from build123d import *

# Parameters (mm, degrees)
MODEL_R                 = 1.600279216
MODEL_R_2               = 1.7
SALIENTE_EXTRUIR2_DEPTH = 3


with BuildPart() as part:
    # Model → Saliente-Extruir2 (new body)
    with BuildSketch(Plane.XY):
        with BuildLine():
            Line((271.351226454, 245.262259879), (270.71262235, 244.623655775))
            Line((270.71262235, 244.623655775), (270.71262235, 230.233550186))
            ThreePointArc((270.71262235, 230.233550186), (271.151962178, 229.172890015), (272.21262235, 228.733550186))
            Line((272.21262235, 228.733550186), (350.217232207, 228.733550186))
            ThreePointArc((350.217232207, 228.733550186), (351.277892379, 229.172890015), (351.717232207, 230.233550186))
            Line((351.717232207, 230.233550186), (351.717232207, 299.235954421))
            ThreePointArc((351.717232208, 299.235954421), (351.277892379, 300.296614592), (350.217232207, 300.735954421))
            Line((350.217232207, 300.735954421), (272.21262235, 300.735954421))
            ThreePointArc((272.21262235, 300.735954421), (271.151962178, 300.296614592), (270.71262235, 299.235954421))
            Line((270.71262235, 299.235954421), (270.71262235, 284.103268217))
            Line((270.71262235, 284.103268217), (271.351226454, 283.464664113))
            Line((271.351226454, 283.464664113), (271.97853318, 283.464664113))
            Line((271.97853318, 283.464664113), (272.77853318, 284.264664113))
            Line((272.77853318, 284.264664113), (276.051226454, 284.264664113))
            Line((276.051226454, 284.264664113), (276.251226454, 284.464664114))
            Line((276.251226454, 284.464664114), (276.251226454, 285.894852324))
            ThreePointArc((276.251226454, 285.894852324), (273.443758266, 287.176917482), (276.239508411, 288.48433854))
            Line((276.239508411, 288.48433854), (276.239508411, 294.917021597))
            ThreePointArc((276.239508411, 294.917021597), (273.696009795, 296.507802753), (276.661013605, 296.964664113))
            Line((276.661013605, 296.964664113), (279.851226454, 296.964664113))
            Line((279.851226454, 296.964664113), (281.651226454, 298.764664113))
            Line((281.651226454, 298.764664113), (341.055836311, 298.764664113))
            Line((341.055836311, 298.764664113), (342.855836311, 296.964664113))
            Line((342.855836311, 296.964664113), (345.9273642, 296.964664113))
            ThreePointArc((345.9273642, 296.964664113), (348.738416986, 297.034405979), (347.268369224, 294.637357529))
            Line((347.268369224, 294.637357529), (347.268369224, 288.812692031))
            ThreePointArc((347.268369224, 288.812692031), (348.543864828, 285.912196427), (345.643369224, 287.187692032))
            Line((345.643369224, 287.187692032), (344.134568969, 287.187692032))
            Line((344.134568969, 287.187692032), (344.134568969, 285.564664113))
            Line((344.134568969, 285.564664113), (344.934568969, 284.764664113))
            Line((344.934568969, 284.764664113), (349.36625565, 284.764664113))
            Line((349.36625565, 284.764664113), (349.86625565, 284.264664113))
            Line((349.86625565, 284.264664113), (349.86625565, 247.072679218))
            Line((349.86625565, 247.072679218), (348.055836311, 245.262259879))
            Line((348.055836311, 245.262259879), (344.855836311, 245.262259879))
            Line((344.855836311, 245.262259879), (344.468087014, 244.877634885))
            Line((344.468087014, 244.877634885), (344.468087014, 231.262259879))
            Line((344.468087014, 231.262259879), (343.968087014, 230.762259879))
            Line((343.968087014, 230.762259879), (278.151226454, 230.762259879))
            Line((278.151226454, 230.762259879), (277.651226454, 231.262259879))
            Line((277.651226454, 231.262259879), (277.651226454, 244.762259879))
            Line((277.651226454, 244.762259879), (277.151226454, 245.262259879))
            Line((277.151226454, 245.262259879), (271.351226454, 245.262259879))
        make_face()
        with Locations((275.263424864, 233.182413169)):
            Circle(MODEL_R, mode=Mode.SUBTRACT)
        with Locations((275.263424864, 242.182078667)):
            Circle(MODEL_R_2, mode=Mode.SUBTRACT)
        with Locations((347.268369224, 233.182413169)):
            Circle(MODEL_R, mode=Mode.SUBTRACT)
        with Locations((347.268369224, 242.182078667)):
            Circle(MODEL_R_2, mode=Mode.SUBTRACT)
    extrude(amount=SALIENTE_EXTRUIR2_DEPTH)


solid = part.part
Can you work these out from the model? Positions are in its coordinate system, mm. A direction names the side the tool comes from. Give positions to 0.01 mm unless a question says otherwise; leave off trailing zeros. Write each loop counter-clockwise with the first axis right and the second up, starting at its lowest first coordinate (ties: lowest second). Pieces come first, ordered by that corner, then holes. Notation, with made-up numbers: M -21.75,3.25 L 36.25,3.25 A18 cw 36.25,29.25 Z; hole C -23,1.25 d5. An arc over 180 degrees is marked long. Answer in a Markdown table with one row per item. Add a question column.
Item 1: Please list where these lines run through material, in increasing order: L1, parallel to Y at x = 302, z = 1.9; L2, parallel to X at y = 286.5, z = 1.65; L3, parallel to Y at x = 342, z = 0.6.
Item 2: We'd pull the mould along X, two halves only. Please class faces 4 (the flat face through (344.468, 238, 1)), 5 (the flat face through (277.651, 238, 1)), 6 (the flat face through (348.974, 246.18, 1.479)), 7 (the flat face through (274, 245.262, 1)): released by +X, released by -X, zero draft, split by the parting line, or undercut.
Item 3: Imagine slicing it at C-C, the plane z = 0.8. State how many separate pieces and enclosed holes the cut face has, plus the area to 3 significant figures.
Item 4: For pin 1 Ø5 at (x, y) = (347.35, 296.24) entering from +Z, with a flat end and sliding along its axis, tell me the tip position at first contact or that it passes through.
Item 5: Imagine slicing it at B-B, the plane y = 267.5. Write out the boundary of the cut face in (x, z).
Item 6: On a 3-axis mill with a long thin cutter (end or side, diameter ignored), from which of +Z, -Z, +X, -X, +Y, -Y can I reach the whole of each face in a straight line? I mean faces 1 (the flat face through (280.739, 297.852, 1.479)), 2 (the flat face through (346, 245.262, 1)), 3 (the flat face through (270.713, 292, 1)). Say none if no direction works.
Item 7: Imagine slicing it at A-A, the plane x = 323. Write out the boundary of the cut face in (y, z), plus the area to 3 significant figures.
Evaluation:
| question | item | result |
|---|---|---|
| 1 | L1 | y = 228.73 to 230.76, 298.76 to 300.74 |
| 1 | L2 | x = 270.71 to 273.59, 344.13 to 345.76, 348.93 to 351.72 |
| 1 | L3 | y = 228.73 to 230.76, 297.82 to 300.74 |
| 2 | face 4 | undercut |
| 2 | face 5 | undercut |
| 2 | face 6 | released by -X |
| 2 | face 7 | zero draft |
| 3 | separate pieces | 1 |
| 3 | enclosed holes | 4 |
| 3 | area | 710 mm² |
| 4 | pin 1 | stops at z = 3 |
| 5 | outline | M 349.87,0 L 351.72,0 L 351.72,3 L 349.87,3 Z |
| 6 | face 1 | +Z, -Z |
| 6 | face 2 | +Z, -Z, -X |
| 6 | face 3 | +Z, -Z, -X, +Y, -Y |
| 7 | outline | M 228.73,0 L 230.76,0 L 230.76,3 L 228.73,3 Z; M 298.76,0 L 300.74,0 L 300.74,3 L 298.76,3 Z |
| 7 | area | 12.0 mm² |
